```python
from build123d import *

# Parameters (mm, degrees)
BOSS_EXTRUDE1_DEPTH = 220
SKETCH2_W           = 31
SKETCH2_H           = 13
CUT_EXTRUDE1_DEPTH  = 10
SKETCH3_R           = 1.55
CUT_EXTRUDE2_DEPTH  = 220
CHAMFER1_SIZE       = 7


with BuildPart() as part:
    # Sketch1 → Boss-Extrude1 (new body)
    with BuildSketch(Plane.XY):
        Polygon((0, 0), (0, 25), (3, 25), (3, 3), (25, 3), (25, 0), align=None)
    extrude(amount=BOSS_EXTRUDE1_DEPTH)

    # Sketch2 → Cut-Extrude1 (cut)
    with BuildSketch(Plane(origin=(3, 0, 0), x_dir=(0, 0, -1), z_dir=(1, 0, 0))):
        with Locations((-110, 9.5)):
            Rectangle(SKETCH2_W, SKETCH2_H)
    extrude(amount=-CUT_EXTRUDE1_DEPTH, mode=Mode.SUBTRACT)

    # Sketch3 → Cut-Extrude2 (cut)
    with BuildSketch(Plane.XZ):
        with Locations((8, 100)):
            Circle(SKETCH3_R)
        with Locations((8, 120)):
            Circle(SKETCH3_R)
        with Locations((8, 215)):
            Circle(SKETCH3_R)
        with Locations((8, 205)):
            Circle(SKETCH3_R)
        with Locations((8, 15)):
            Circle(SKETCH3_R)
        with Locations((8, 5)):
            Circle(SKETCH3_R)
        with Locations((20, 120)):
            Circle(SKETCH3_R)
        with Locations((20, 100)):
            Circle(SKETCH3_R)
        with Locations((20, 15)):
            Circle(SKETCH3_R)
        with Locations((20, 205)):
            Circle(SKETCH3_R)
    extrude(amount=-CUT_EXTRUDE2_DEPTH, mode=Mode.SUBTRACT)

    # Chamfer1
    chamfer1_edges = [part.edges().sort_by_distance(p)[0] for p in [
        (1.5, 25, 220),
        (1.5, 25, 0),
    ]]
    chamfer(chamfer1_edges, length=CHAMFER1_SIZE)


solid = part.part
```
Source: CAD feature listing. Evaluate the final solid. Frame: model axes, mm. A direction names the side the tool comes from. Coordinates: 2 decimals unless noted, no trailing zeros. Write each loop counter-clockwise with the first axis right and the second up, starting at its lowest first coordinate (ties: lowest second). Pieces come first, ordered by that corner, then holes. Notation, with made-up numbers: M 51,5 L 107,5 A19 cw 107,23 Z; hole C -27,40.25 d2. An arc over 180 degrees is marked long. Answer as a JSON object with one key per item and string values.
1. Cut plane B-B on z = 79.5. Output: boundary loops of the cut face in (x, y), plus the area to 3 significant figures.
Evaluation:
{"outline": "M 0,0 L 25,0 L 25,3 L 3,3 L 3,25 L 0,25 Z", "area": "141 mm^2"}
2. Cut plane A-A on y = 9.25. Output: boundary loops of the cut face in (x, z), plus the area to 3 significant figures.
Evaluation:
{"outline": "M 0,0 L 3,0 L 3,94.5 L 0,94.5 Z; M 0,125.5 L 3,125.5 L 3,220 L 0,220 Z", "area": "567 mm^2"}
3. Ray query, L1, parallel to X at y = 2.1, z = 100; L2, parallel to Z at x = 20, y = 0.75; L3, parallel to X at y = 1.2, z = 215. Return the intervals inside material, ascending.
Evaluation:
{"L1": "0 to 6.45, 9.55 to 18.45, 21.55 to 25", "L2": "0 to 13.45, 16.55 to 98.45, 101.55 to 118.45, 121.55 to 203.45, 206.55 to 220", "L3": "0 to 6.45, 9.55 to 25"}
4. Contact query for flat-ended pins moving along their axis: P1, Ø1.5, axis at y = 20.5, z = 158, coming from the +X side; P2, Ø4, axis at x = 8, z = 215, coming from the +Y side; P3, Ø1.9, axis at x = 8, z = 100, coming from the -Y side. Output: stop coordinate, or through.
Evaluation:
{"P1": "x = 3", "P2": "y = 3", "P3": "through"}
5. Access query for faces 1 (the flat face through (3, 17, 108)), 2 (the flat face through (1, 22, 4)). Directions: +Z, -Z, +X, -X, +Y, -Y. A direction counts if a zero-diameter tool reaches every point of the face in a straight line with its end or side. Return the directions, or none.
Evaluation:
{"face 1": "+Z, -Z, +X, +Y", "face 2": "-Z, +X, -X, +Y"}
